```python
from build123d import *

# Parameters (mm, degrees)
F1_DEPTH = 48


with BuildPart() as f1:
    # F0 (on Front) → F1 (new body)
    with BuildSketch(Plane.XZ):
        Polygon((0, 14.997751), (0, 0), (9.975666, 0), (18.991238, 9.989237), (18.991238, 11.026427), (20, 11.026427), (20.985832, 11.026427), (20.985832, 10.069021), (30.001402, 0), (40, 0), (40, 15.031243), (34.019962, 15.031243), (34.019962, 25.028992), (40, 25.028992), (40, 40), (35.052698, 40), (21.043338, 25.028992), (21.043338, 23.991385), (20.042421, 23.991385), (19.001365, 23.991385), (19.001365, 25.028992), (5.032144, 40), (0, 40), (0, 24.992259), (5.982323, 24.992259), (5.982323, 14.997751), align=None)
    extrude(amount=-F1_DEPTH)


solid = f1.part
```
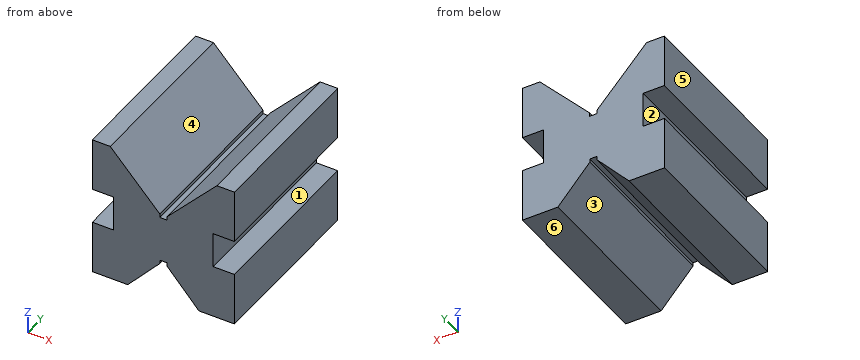
Model file for the job. Use its own axes, mm. Face numbers are marked on the shaded views. A direction names the side the tool comes from. Give positions to 0.01 mm unless a question says otherwise; leave off trailing zeros. Order: outer loops, then holes, each group sorted by start corner. A loop starts at its lowest first (then second) coordinate and runs counter-clockwise, first axis right, second up.
1) Saw through at B-B, the plane z = 36. Write the cut outline in (x, y), then the cut area to 3 significant figures.
2) Saw through at D-D, the plane z = 16. Write the cut outline in (x, y).
3) Wall check: probe 1 along Z at (x, y) = (36.5, 16); probe 2 along X at (y, z) = (11, 35.5); probe 3 along X at (y, z) = (27, 35). Give the ranges that are in metal, low to high.
4) Saw through at C-C, the plane y = 3.5. Write the cut outline in (x, z).
5) Pin check, flat tips, straight feed: pin 1 (3 mm diameter, centred on y = 30, z = 19, fed in from -X); pin 2 (1 mm diameter, centred on x = 4.5, z = 18, fed in from -Y); pin 3 (1.6 mm diameter, centred on x = 19.5, y = 26, fed in from +Z); pin 4 (0.6 mm diameter, centred on x = 20, y = 15, fed in from -Z). Stop position of each tip, or through.
6) Mould opens along X. For the marked faces 4, 5 and 6 say: +X half, -X half, draft (parallel to the pull), parting line (faces both ways), or undercut.
7) Saw through at A-A, the plane x = 3. Write the cut outline in (y, z).
8) 3-axis set-ups, long thin cutter, end or side, ignore diameter. For the marked faces 1, 2 and 3: which of +Z, -Z, +X, -X, +Y, -Y reach the whole face in a straight line?
Computed:
1. outline: (0, 0) - (8.76, 0) - (8.76, 48) - (0, 48) - close; (31.31, 0) - (40, 0) - (40, 48) - (31.31, 48) - close
1. area: 838 mm2
2. outline: (5.98, 0) - (34.02, 0) - (34.02, 48) - (5.98, 48) - close
3. probe 1: z = 0 to 15.03, 25.03 to 40
3. probe 2: x = 0 to 9.23, 30.84 to 40
3. probe 3: x = 0 to 9.7, 30.37 to 40
4. outline: (0, 0) - (9.98, 0) - (18.99, 9.99) - (18.99, 11.03) - (20.99, 11.03) - (20.99, 10.07) - (30, 0) - (40, 0) - (40, 15.03) - (34.02, 15.03) - (34.02, 25.03) - (40, 25.03) - (40, 40) - (35.05, 40) - (21.04, 25.03) - (21.04, 23.99) - (19, 23.99) - (19, 25.03) - (5.03, 40) - (0, 40) - (0, 24.99) - (5.98, 24.99) - (5.98, 15) - (0, 15) - close
5. pin 1: stops at x = 5.98
5. pin 2: passes through
5. pin 3: stops at z = 25.35
5. pin 4: stops at z = 11.03
6. face 4: undercut
6. face 5: -X half
6. face 6: draft
7. outline: (0, 0) - (48, 0) - (48, 15) - (0, 15) - close; (0, 24.99) - (48, 24.99) - (48, 40) - (0, 40) - close
8. face 1: +X, +Y, -Y
8. face 2: -X, +Y, -Y
8. face 3: -Z, +Y, -Y
